```python
from build123d import *

# Parameters (mm, degrees)
SKETCH1_W           = 20
SKETCH1_H           = 20
BOSS_EXTRUDE1_DEPTH = 10
SKETCH_Z_R          = 6
CUT_EXTRUDE1_DEPTH  = 16
SKETCH_Y_R          = 6
CUT_EXTRUDE2_DEPTH  = 16
SKETCH_X_R          = 6
CUT_EXTRUDE3_DEPTH  = 16
SKETCH32_W          = 5.4
SKETCH32_H          = 3
SKETCH32_W_2        = 3
SKETCH32_H_2        = 5.4
CON_DEPTH           = 2.9
CIRPATTERN5_COUNT   = 2
CIRPATTERN5_ANGLE   = 270
CIRPATTERN9_COUNT   = 2
CIRPATTERN9_ANGLE   = 90


with BuildPart() as part:
    # Sketch1 → Boss-Extrude1 (new, symmetric)
    with BuildSketch(Plane(origin=(0, 0, 0), x_dir=(1, 0, 0), z_dir=(0, 1, 0))):
        Rectangle(SKETCH1_W, SKETCH1_H)
    extrude(amount=BOSS_EXTRUDE1_DEPTH, both=True)

    # Sketch Z → Cut-Extrude1 (cut)
    with BuildSketch(Plane.XY.offset(10)):
        Circle(SKETCH_Z_R)
    extrude(amount=-CUT_EXTRUDE1_DEPTH, mode=Mode.SUBTRACT)

    # Sketch Y → Cut-Extrude2 (cut)
    with BuildSketch(Plane(origin=(0, 10, 0), x_dir=(1, 0, 0), z_dir=(0, 1, 0))):
        with Locations(Location((0, 0, 0), (0, 0, 270))):
            Circle(SKETCH_Y_R)
    extrude(amount=-CUT_EXTRUDE2_DEPTH, mode=Mode.SUBTRACT)

    # Sketch X → Cut-Extrude3 (cut)
    with BuildSketch(Plane(origin=(10, 0, 0), x_dir=(0, 0, -1), z_dir=(1, 0, 0))):
        Circle(SKETCH_X_R)
    extrude(amount=-CUT_EXTRUDE3_DEPTH, mode=Mode.SUBTRACT)

    # Sketch23 → CSK for M6 Flat Head Machine Screw23 (revolve, cut)
    with BuildSketch(Plane(origin=(-6, 0, 0), x_dir=(0, 0, -1), z_dir=(0, 1, 0))):
        Polygon((0, 0), (0, 4), (3, 4), (3, 3), (6, 0), align=None)
    revolve(axis=Axis((0.35, 0, 0), (-1, 0, 0)), mode=Mode.SUBTRACT)

    # Sketch24 → CSK for M6 Flat Head Machine Screw24 (revolve, cut)
    with BuildSketch(Plane(origin=(0, 0, -6), x_dir=(0, -1, 0), z_dir=(1, 0, 0))):
        Polygon((0, 0), (0, 4), (3, 4), (3, 3), (6, 0), align=None)
    revolve(axis=Axis((0, 0, 0.35), (0, 0, -1)), mode=Mode.SUBTRACT)

    # Sketch26 → CSK for M6 Flat Head Machine Screw25 (revolve, cut)
    with BuildSketch(Plane(origin=(0, -6, 0), x_dir=(0, 0, 1), z_dir=(1, 0, 0))):
        Polygon((0, 0), (0, 4), (3, 4), (3, 3), (6, 0), align=None)
    revolve(axis=Axis((0, 0.35, 0), (0, -1, 0)), mode=Mode.SUBTRACT)

    # Sketch32 → con (add, symmetric)
    with BuildSketch(Plane.XY):
        Polygon((-10, -10), (-10, -4.6), (-13, -4.6), (-13, -11), (-11, -13), (-4.6, -13), (-4.6, -10), align=None)
        with Locations((7.3, -11.5)):
            Rectangle(SKETCH32_W, SKETCH32_H)
        with Locations((-11.5, 7.3)):
            Rectangle(SKETCH32_W_2, SKETCH32_H_2)
    con = extrude(amount=CON_DEPTH, both=True)

    # CirPattern5: con ×2 about axis
    cirpattern5_axis = Axis((0, 0, 0), (0, 1, 0))
    for i in range(1, CIRPATTERN5_COUNT):
        add(con.rotate(cirpattern5_axis, i * CIRPATTERN5_ANGLE / (CIRPATTERN5_COUNT - 1)))

    # CirPattern9: con ×2 about axis
    cirpattern9_axis = Axis((0, 0, 0), (1, 0, 0))
    for i in range(1, CIRPATTERN9_COUNT):
        add(con.rotate(cirpattern9_axis, i * CIRPATTERN9_ANGLE / (CIRPATTERN9_COUNT - 1)))


solid = part.part
```
Model file for the job. Use its own axes, mm. A direction names the side the tool comes from. Give positions to 0.01 mm unless a question says otherwise; leave off trailing zeros. Order: outer loops, then holes, each group sorted by start corner. A loop starts at its lowest first (then second) coordinate and runs counter-clockwise, first axis right, second up.
1) Saw through at A-A, the plane y = -11.5. Write the cut outline in (x, z).
2) Saw through at D-D, the plane x = -10.5. Write the cut outline in (y, z), then the cut area to 3 significant figures.
3) Mould opens along Z. For faces 6 (the flat face through (-12, 0, -12)), 7 (the cylindrical face through (4.258, -5.443, -4.227)), 8 (the cylindrical face through (4.06, 7.8, -4.42)), 9 (the flat face through (0, -13, -8)) say: +Z half, -Z half, draft (parallel to the pull), parting line (faces both ways), or undercut.
4) Pin check, flat tips, straight feed: pin 1 (9 mm diameter, centred on x = -8.5, y = -9.5, fed in from -Z); pin 2 (2 mm diameter, centred on y = 4.5, z = -4.5, fed in from -X); pin 3 (5 mm diameter, centred on x = 0, z = 0, fed in from -Y); pin 4 (1.5 mm diameter, centred on y = -12, z = -1.5, fed in from -X). Stop position of each tip, or through.
5) 3-axis set-ups, long thin cutter, end or side, ignore diameter. For faces 1 (the flat face through (-12, 2.9, 7)), 2 (the flat face through (0, -4.6, -11)), 3 (the flat face through (4.6, -12, 0)), 4 (the flat face through (2.9, 7, -12)), 5 (the cylindrical face through (4.227, -5.443, 4.258)): which of +Z, -Z, +X, -X, +Y, -Y reach the whole face in a straight line?
6) Saw through at B-B, the plane x = 8.25. Write the cut outline in (y, z).
7) Wall check: probe 1 along Z at (x, y) = (-10.5, 0); probe 2 along Z at (x, y) = (-4.25, 8.75); probe 3 along X at (y, z) = (-9.35, 0). Give the ranges that are in metal, low to high.
Computed:
1. outline: (-12.5, -2.9) - (-4.6, -2.9) - (-4.6, 2.9) - (-12.5, 2.9) - close; (-2.9, -12.5) - (2.9, -12.5) - (2.9, -4.6) - (-2.9, -4.6) - close; (-2.9, 4.6) - (2.9, 4.6) - (2.9, 10) - (-2.9, 10) - close; (4.6, -2.9) - (10, -2.9) - (10, 2.9) - (4.6, 2.9) - close
2. outline: (-13, -2.9) - (-4.6, -2.9) - (-4.6, 2.9) - (-13, 2.9) - close; (-2.9, -13) - (2.9, -13) - (2.9, -4.6) - (-2.9, -4.6) - close; (-2.9, 4.6) - (2.9, 4.6) - (2.9, 10) - (-2.9, 10) - close; (4.6, -2.9) - (10, -2.9) - (10, 2.9) - (4.6, 2.9) - close
2. area: 160 mm2
3. face 6: -Z half
3. face 7: undercut
3. face 8: undercut
3. face 9: draft
4. pin 1: stops at z = -10
4. pin 2: stops at x = -10
4. pin 3: passes through
4. pin 4: stops at x = -12.75
5. face 1: +Z, -Z, -X, +Y
5. face 2: -Z, +X, -X
5. face 3: +Z, -Z, -Y
5. face 4: -Z, +X, +Y, -Y
5. face 5: +Y
6. outline: (-13, -2.9) - (-10, -2.9) - (-10, -10) - (-2.9, -10) - (-2.9, -13) - (2.9, -13) - (2.9, -10) - (10, -10) - (10, 10) - (-10, 10) - (-10, 2.9) - (-13, 2.9) - close; hole circle Ø12 at (0, 0)
7. probe 1: z = -13 to -4.6, 4.6 to 10
7. probe 2: z = -10 to -4.24, 4.24 to 10
7. probe 3: x = -13 to -3, 3 to 10
